Read the model definition and answer for the solid it produces. Units are mm, in the model's axes. A direction names the side the tool comes from. Round coordinates to 2 decimals unless told otherwise and drop trailing zeros. Order: outer loops, then holes, each group sorted by start corner. A loop starts at its lowest first (then second) coordinate and runs counter-clockwise, first axis right, second up. Notation, with made-up numbers: (-22, 35) - (5, 35) arc R19 ccw to (5, 39) - close; hole circle Ø5 at (64, -1). An arc over 180 degrees is marked (long way). Answer as a JSON object with one key per item and string values. Group by question number.
Q1. A cutting plane is placed at A-A on x = -14.5. Determine the outline of the cut face in (y, z).
Q2. A cutting plane is placed at B-B on x = -7.7. Determine the outline of the cut face in (y, z), and give its area (3 significant figures).
Q3. A tool of negligible diameter and unlimited length cuts with its end or side. For faces 1 (the cylindrical face through (-6.53, -17.19, 0.59)), 2 (the cylindrical face through (-11.27, -12.18, 0.59)), from which of +Z, -Z, +X, -X, +Y, -Y can it reach the whole face along a straight path? Write none if from no direction.
Q4. The mould has two halves that part along X. Classify faces 3 (the cylindrical face through (11.2, -12.2, 0.6)), 4 (the flat face through (0, 16, 0)), 5 (the cylindrical face through (-0.717, 18.986, 0.592)), 6 (the cylindrical face through (5.86, -12.39, 0.59)): pulls with the +X half, pulls with the -X half, needs draft (parallel to the pull), parting line crosses it, or undercut.
Q5. A cutting plane is placed at D-D on z = 0.95. Determine the outline of the cut face in (x, y).
Q6. A cutting plane is placed at C-C on y = -8. Determine the outline of the cut face in (x, z).
Q7. Consider line 1 (Y direction, x = -7.7, z = 0.7); line 2 (X direction, y = -15, z = 0.25); line 3 (X direction, y = -0.5, z = 0.85). Determine where each line is inside the solid, lowest interval first.
```python
from build123d import *

# Parameters (mm, degrees)
SKETCH_1_R      = 1.25
EXTRUDE_1_DEPTH = 1.2


with BuildPart() as part:
    # Эскиз1 → Бобышка-Вытянуть1 (new body)
    with BuildSketch(Plane.XY):
        with BuildLine():
            Line((-5.160647232, -15.284063293), (-5.429258829, -16.027548533))
            ThreePointArc((-5.429258829, -16.027548533), (-6.550261386, -17.197940013), (-8.170291571, -17.153609989))
            ThreePointArc((-8.170291571, -17.153609989), (0, 19), (8.170291571, -17.153609989))
            ThreePointArc((8.170291571, -17.153609989), (6.550261386, -17.197940013), (5.429258829, -16.027548533))
            Line((5.429258829, -16.027548533), (5.160647232, -15.284063293))
            ThreePointArc((5.160647232, -15.284063293), (5.893948192, -12.359596142), (8.879298744, -11.937789906))
            ThreePointArc((8.879298744, -11.937789906), (11.233706363, -12.19050777), (13.210178389, -10.88641426))
            ThreePointArc((13.210178389, -10.88641426), (0, 15.5), (-13.210178389, -10.88641426))
            ThreePointArc((-13.210178389, -10.88641426), (-11.233706363, -12.19050777), (-8.879298744, -11.937789906))
            ThreePointArc((-8.879298744, -11.937789906), (-5.893948192, -12.359596142), (-5.160647232, -15.284063293))
        make_face()
        with Locations((-7.7, -14.366627997)):
            Circle(SKETCH_1_R, mode=Mode.SUBTRACT)
        with Locations((7.7, -14.366627997)):
            Circle(SKETCH_1_R, mode=Mode.SUBTRACT)
    extrude(amount=EXTRUDE_1_DEPTH)


solid = part.part
```
Result set:
{
 "1": {"outline": "(-12.28, 0) - (-8.87, 0) - (-8.87, 1.2) - (-12.28, 1.2) - close; (6.87, 0) - (12.28, 0) - (12.28, 1.2) - (6.87, 1.2) - close"},
 "2": {"outline": "(-17.31, 0) - (-15.62, 0) - (-15.62, 1.2) - (-17.31, 1.2) - close; (-13.12, 0) - (-11.67, 0) - (-11.67, 1.2) - (-13.12, 1.2) - close; (13.59, 0) - (17.37, 0) - (17.37, 1.2) - (13.59, 1.2) - close", "area": "8.30 mm²"},
 "3": {"face 1": "+Z, -Z, -Y", "face 2": "+Z, -Z"},
 "4": {"face 3": "undercut", "face 4": "needs draft", "face 5": "parting line crosses it", "face 6": "undercut"},
 "5": {"outline": "(-13.21, -10.89) arc R16.5 cw (long way) to (13.21, -10.89) arc R3.5 cw to (8.88, -11.94) arc R2.7 ccw to (5.16, -15.28) - (5.43, -16.03) arc R2 ccw to (8.17, -17.15) arc R19 ccw (long way) to (-8.17, -17.15) arc R2 ccw to (-5.43, -16.03) - (-5.16, -15.28) arc R2.7 ccw to (-8.88, -11.94) arc R3.5 cw to start; hole circle Ø2.5 at (-7.7, -14.37); hole circle Ø2.5 at (7.7, -14.37)"},
 "6": {"outline": "(-17.23, 0) - (-14.94, 0) - (-14.94, 1.2) - (-17.23, 1.2) - close; (14.94, 0) - (17.23, 0) - (17.23, 1.2) - (14.94, 1.2) - close"},
 "7": {"line 1": "y = -17.31 to -15.62, -13.12 to -11.67, 13.59 to 17.37", "line 2": "x = -11.66 to -8.78, -6.62 to -5.08, 5.08 to 6.62, 8.78 to 11.66", "line 3": "x = -18.99 to -16.49, 16.49 to 18.99"}
}
